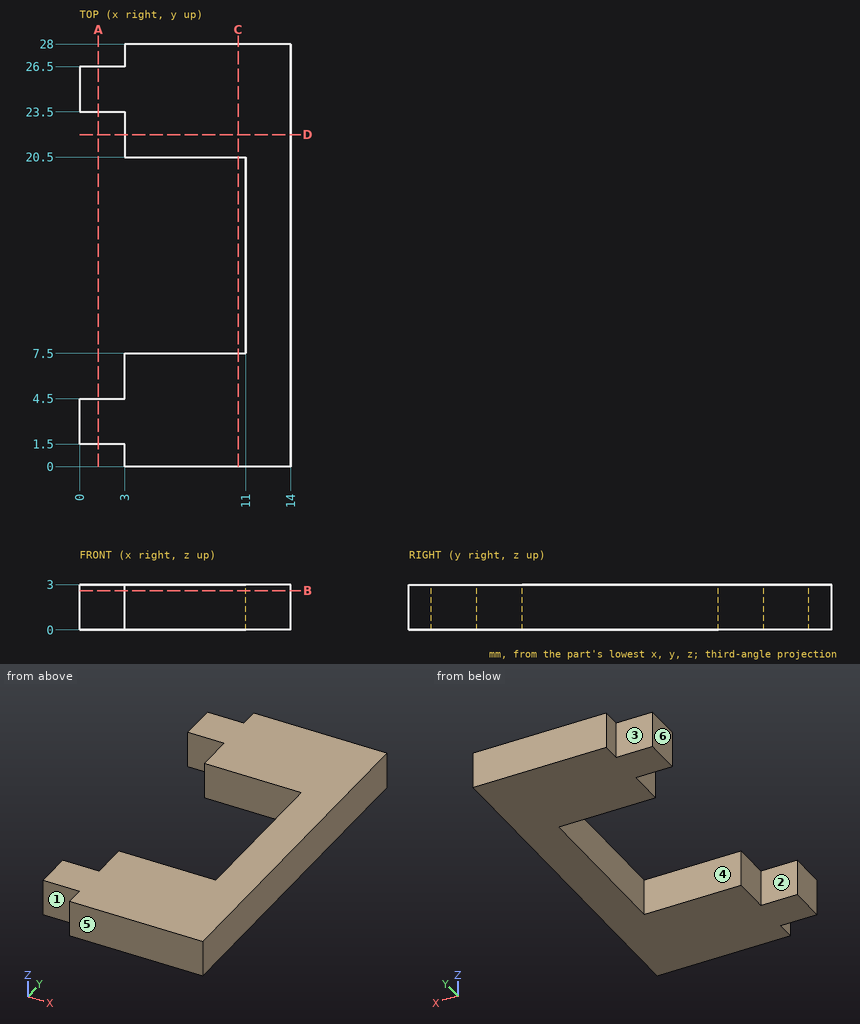
Study the drawing (mm; zero at the part's minimum x, y, z) and answer. A direction names the side the tool comes from. Round coordinates to 2 decimals unless told otherwise and drop trailing zeros. Write each loop counter-clockwise with the first axis right and the second up, starting at its lowest first coordinate (ties: lowest second). Pieces come first, ordered by that corner, then holes. Notation, with made-up numbers: (14.25, 15.5) -> (46.25, 15.5) arc R19 ccw to (46.25, 29.5) -> close; hole circle Ø7 at (64, 87.5). An arc over 180 degrees is marked (long way). Write item = value, one per line.
1) Given pin 1 (0.9 mm diameter, centred on y = 22, z = 2, fed in from -X); pin 2 (1.6 mm diameter, centred on y = 27, z = 2, fed in from -X); pin 3 (1.5 mm diameter, centred on x = 1.5, z = 1, fed in from +Y); pin 4 (0.9 mm diameter, centred on x = 2, z = 1, fed in from -Y), each flat-ended and moving along its own axis, determine where each tip first touches the part or whether it passes through.
Check values:
pin_1 = 3
pin_2 = 0
pin_3 = 26.5
pin_4 = 1.5
2) Section B-B on z = 2.6 is taken. Write down the section's boundary in (x, y).
Check values:
outline = (0, 1.5) -> (3, 1.5) -> (3, 0) -> (14, 0) -> (14, 28) -> (3, 28) -> (3, 26.5) -> (0, 26.5) -> (0, 23.5) -> (3, 23.5) -> (3, 20.5) -> (11, 20.5) -> (11, 7.5) -> (3, 7.5) -> (3, 4.5) -> (0, 4.5) -> close
3) Straight lines are drawn through the part: line 1 along Y through (x, z) = (10.75, 2.1); line 2 along Y through (x, z) = (2.25, 2); line 3 along X through (y, z) = (23, 2.45). For each, find the intervals that lie inside material, in ascending order. Write a range as [from, to].
Check values:
line_1 = [0, 7.5], [20.5, 28]
line_2 = [1.5, 4.5], [23.5, 26.5]
line_3 = [3, 14]
4) Which of the six approach directions +Z, -Z, +X, -X, +Y, -Y give full straight-line access (tool end or side, diameter ignored) to the marked faces 1, 2 and 3?
Check values:
face_1 = +Z, -Z, -X, -Y
face_2 = +Z, -Z, -X
face_3 = +Z, -Z, -X, +Y
5) Section D-D on y = 22 is taken. Write down the section's boundary in (x, z).
Check values:
outline = (3, 0) -> (14, 0) -> (14, 3) -> (3, 3) -> close
6) Section C-C on x = 10.5 is taken. Write down the section's boundary in (y, z).
Check values:
outline = (0, 0) -> (7.5, 0) -> (7.5, 3) -> (0, 3) -> close; (20.5, 0) -> (28, 0) -> (28, 3) -> (20.5, 3) -> close
7) Section A-A on x = 1.25 is taken. Write down the section's boundary in (y, z), plus the area to 3 significant figures.
Check values:
outline = (1.5, 0) -> (4.5, 0) -> (4.5, 3) -> (1.5, 3) -> close; (23.5, 0) -> (26.5, 0) -> (26.5, 3) -> (23.5, 3) -> close
area = 18.0 mm²
8) For a pull along Y with two mould halves and no side action, classify the marked faces 4, 5 and 6 as released by +Y, released by -Y, zero draft, split by the parting line, or undercut.
Check values:
face_4 = undercut
face_5 = released by -Y
face_6 = zero draft
